```python
from build123d import *

# Parameters (mm, degrees)
PAD_DEPTH          = 9
SKETCH001_W        = 26.1
SKETCH001_H        = 34.4
POCKET_DEPTH       = 3
SKETCH002_R        = 22.22
PAD001_DEPTH       = 3
SKETCH003_R        = 24.44
PAD002_DEPTH       = 3
SKETCH004_R        = 26.6
PAD003_DEPTH       = 3
SKETCH005_R        = 28
PAD004_DEPTH       = 3
SKETCH006_R        = 29
PAD005_DEPTH       = 3
SKETCH007_R        = 29
PAD006_DEPTH       = 3
SKETCH008_R        = 29
PAD007_DEPTH       = 3
SKETCH009_W        = 17
SKETCH009_H        = 24
POCKET001_DEPTH    = 3
SKETCH010_W        = 16
SKETCH010_H        = 9
POCKET002_DEPTH    = 7
SKETCH011_W        = 20
SKETCH011_H        = 9
POCKET003_DEPTH    = 3
SKETCH012_R        = 1.25
POCKET004_DEPTH    = 270.433943
POLARPATTERN_COUNT = 6
SKETCH013_W        = 3
SKETCH013_H        = 38
POCKET005_DEPTH    = 3
SKETCH014_W        = 3
SKETCH014_H        = 6
POCKET006_DEPTH    = 6
SKETCH015_W        = 10.05
SKETCH015_H        = 6
POCKET007_DEPTH    = 3
FILLET_R           = 4


with BuildPart() as part:
    # Sketch → Pad (new body)
    with BuildSketch(Plane.XY):
        Polygon((44, 0), (22, 38.105118), (-22, 38.105118), (-44, 0), (-22, -38.105118), (22, -38.105118), align=None)
    extrude(amount=PAD_DEPTH)

    # Sketch001 (on Face8 of Pad) → Pocket (cut)
    with BuildSketch(Plane.XY.offset(9)):
        with Locations((0, -13.905118)):
            Rectangle(SKETCH001_W, SKETCH001_H)
    extrude(amount=-POCKET_DEPTH, mode=Mode.SUBTRACT)

    # Sketch002 (on Face5 of Pocket) → Pad001 (join)
    with BuildSketch(Plane.XY.offset(9)):
        Polygon((22, 38.105118), (-22, 38.105118), (-44, 0), (-22, -38.105118), (22, -38.105118), (44, 0), align=None)
        Circle(SKETCH002_R, mode=Mode.SUBTRACT)
    extrude(amount=PAD001_DEPTH)

    # Sketch003 (on Face14 of Pad001) → Pad002 (join)
    with BuildSketch(Plane.XY.offset(12)):
        Polygon((40, 0), (20, 34.641016), (-20, 34.641016), (-40, 0), (-20, -34.641016), (20, -34.641016), align=None)
        Circle(SKETCH003_R, mode=Mode.SUBTRACT)
    extrude(amount=PAD002_DEPTH)

    # Sketch004 (on Face21 of Pad002) → Pad003 (join)
    with BuildSketch(Plane.XY.offset(15)):
        Polygon((41, 0), (20.5, 35.507042), (-20.5, 35.507042), (-41, 0), (-20.5, -35.507042), (20.5, -35.507042), align=None)
        Circle(SKETCH004_R, mode=Mode.SUBTRACT)
    extrude(amount=PAD003_DEPTH)

    # Sketch005 (on Face28 of Pad003) → Pad004 (join)
    with BuildSketch(Plane.XY.offset(18)):
        Polygon((19, 32.908965), (-19, 32.908965), (-38, 0), (-19, -32.908965), (19, -32.908965), (38, 0), align=None)
        Circle(SKETCH005_R, mode=Mode.SUBTRACT)
    extrude(amount=PAD004_DEPTH)

    # Sketch006 (on Face35 of Pad004) → Pad005 (join)
    with BuildSketch(Plane.XY.offset(21)):
        Polygon((39, 0), (19.5, 33.774991), (-19.5, 33.774991), (-39, 0), (-19.5, -33.774991), (19.5, -33.774991), align=None)
        Circle(SKETCH006_R, mode=Mode.SUBTRACT)
    extrude(amount=PAD005_DEPTH)

    # Sketch007 (on Face42 of Pad005) → Pad006 (join)
    with BuildSketch(Plane.XY.offset(24)):
        Polygon((36, 0), (18, 31.176915), (-18, 31.176915), (-36, 0), (-18, -31.176915), (18, -31.176915), align=None)
        Circle(SKETCH007_R, mode=Mode.SUBTRACT)
    extrude(amount=PAD006_DEPTH)

    # Sketch008 (on Face49 of Pad006) → Pad007 (join)
    with BuildSketch(Plane.XY.offset(27)):
        Polygon((37, 0), (18.5, 32.04294), (-18.5, 32.04294), (-37, 0), (-18.5, -32.04294), (18.5, -32.04294), align=None)
        Circle(SKETCH008_R, mode=Mode.SUBTRACT)
    extrude(amount=PAD007_DEPTH)

    # Sketch009 (on Face74 of Pad007) → Pocket001 (cut)
    with BuildSketch(Plane.XY.offset(6)):
        with Locations((0, -8.705118)):
            Rectangle(SKETCH009_W, SKETCH009_H)
    extrude(amount=-POCKET001_DEPTH, mode=Mode.SUBTRACT)

    # Sketch010 (on Face12 of Pocket001) → Pocket002 (cut)
    with BuildSketch(Plane.XZ.offset(38.105118)):
        with Locations((0, 7.5)):
            Rectangle(SKETCH010_W, SKETCH010_H)
    extrude(amount=-POCKET002_DEPTH, mode=Mode.SUBTRACT)

    # Sketch011 (on Face40 of Pocket002) → Pocket003 (cut)
    with BuildSketch(Plane.XY.offset(9)):
        with Locations((0, 17.72)):
            Rectangle(SKETCH011_W, SKETCH011_H)
    extrude(amount=-POCKET003_DEPTH, mode=Mode.SUBTRACT)

    # Sketch012 (on Face93 of Pocket003) → Pocket004 (cut, through all)
    with BuildSketch(Plane.XY.offset(30)):
        with Locations((-32.33, 0)):
            Circle(SKETCH012_R)
    pocket004 = extrude(amount=-POCKET004_DEPTH, mode=Mode.SUBTRACT)

    # PolarPattern: Pocket004 ×6 about axis
    polarpattern_axis = Axis((0, 0, 30), (0, 0, 1))
    for i in range(1, POLARPATTERN_COUNT):
        add(pocket004.rotate(polarpattern_axis, i * 360 / POLARPATTERN_COUNT), mode=Mode.SUBTRACT)

    # Sketch013 (on Face45 of PolarPattern) → Pocket005 (cut)
    with BuildSketch(Plane.XY.offset(6)):
        with Locations((-11.55, -12.105118)):
            Rectangle(SKETCH013_W, SKETCH013_H)
    extrude(amount=-POCKET005_DEPTH, mode=Mode.SUBTRACT)

    # Sketch014 (on Face58 of Pocket005) → Pocket006 (cut)
    with BuildSketch(Plane.XY.offset(9)):
        with Locations((-11.55, 6.294882)):
            Rectangle(SKETCH014_W, SKETCH014_H)
    extrude(amount=-POCKET006_DEPTH, mode=Mode.SUBTRACT)

    # Sketch015 (on Face58 of Pocket006) → Pocket007 (cut)
    with BuildSketch(Plane.XY.offset(9)):
        with Locations((-5.025, 6.294882)):
            Rectangle(SKETCH015_W, SKETCH015_H)
    extrude(amount=-POCKET007_DEPTH, mode=Mode.SUBTRACT)

    # Fillet
    fillet_edges = [part.edges().sort_by_distance(p)[0] for p in [
        (22, -38.105118, 4.5),
        (44, 0, 4.5),
        (22, 38.105118, 4.5),
        (-22, 38.105118, 4.5),
        (-44, 0, 4.5),
        (-22, -38.105118, 4.5),
    ]]
    fillet(fillet_edges, radius=FILLET_R)


solid = part.part
```
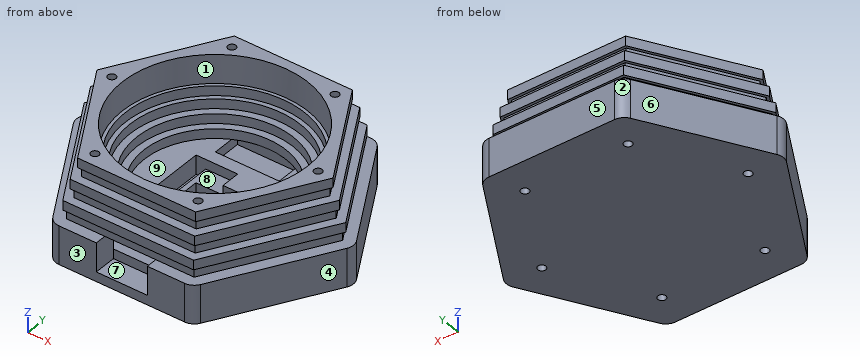
Check sheet for the modelled part. Datum: model origin and axes. Units: mm. Face numbers are marked on the shaded views. A direction names the side the tool comes from. Round coordinates to 2 decimals unless told otherwise and drop trailing zeros. Order: outer loops, then holes, each group sorted by start corner. A loop starts at its lowest first (then second) coordinate and runs counter-clockwise, first axis right, second up. Notation, with made-up numbers: (62.5, -29.75) - (111.5, -29.75) arc R36 ccw to (111.5, 4.25) - close; hole circle Ø9 at (-31.5, 44.5). An arc over 180 degrees is marked (long way). Answer as CSV lines item,"result". Start each with the question number.
1) Section check B-B (z = 4). Give the number of separate pieces and of enclosed holes in the cut face, then the cut area to 3 significant figures.
2) Scan lines: probe 1 along Z at (x, y) = (-8, 32); probe 2 along Y at (x, z) = (15.5, 23.75) (3 decimals); probe 3 along Z at (x, y) = (9, -33). Record each from-to range of solid material in increasing order.
3) Section check D-D (x = -35). Record the cut outline in (y, z), then the cut area to 3 significant figures.
4) Draft check along X on the marked faces 1, 2, 3 and 4. Enter one of: +X half, -X half, draft (parallel to the pull), parting line (faces both ways), or undercut.
5) Section check C-C (z = 19). Record the cut outline in (x, y) (3 decimals), then the cut area to 3 significant figures.
6) Tool access check on the marked faces 5, 6, 7, 8 and 9. Record the directions out of +Z, -Z, +X, -X, +Y, -Y that give a thin tool (end or side, any length) a straight path to the whole face; none if there is none.
7) Depth check by flat-ended pin: pin 1 (6 mm diameter, centred on x = 29.5, z = 16, fed in from -Y); pin 2 (10 mm diameter, centred on y = -13.5, z = 12, fed in from -X); pin 3 (0.9 mm diameter, centred on x = -6.5, z = 13.5, fed in from +Y). Enter the tip coordinate at first touch or a pass-through.
Determined:
1,separate pieces,"1"
1,enclosed holes,"8"
1,area,"4,350 mm^2"
2,probe 1,"0 to 24, 27 to 30"
2,probe 2,"-33.775 to -29.057, -26.94 to -24.51, 24.51 to 26.94, 29.057 to 33.775"
2,probe 3,"0 to 18, 21 to 24"
3,outline,"(-15.59, 0) - (15.59, 0) - (15.59, 12) - (8.66, 12) - (8.66, 15) - (10.39, 15) - (10.39, 18) - (5.2, 18) - (5.2, 21) - (6.93, 21) - (6.93, 24) - (1.73, 24) - (1.73, 27) - (3.46, 27) - (3.46, 30) - (-3.46, 30) - (-3.46, 27) - (-1.73, 27) - (-1.73, 24) - (-6.93, 24) - (-6.93, 21) - (-5.2, 21) - (-5.2, 18) - (-10.39, 18) - (-10.39, 15) - (-8.66, 15) - (-8.66, 12) - (-15.59, 12) - close"
3,area,"592 mm^2"
4,face 1,"undercut"
4,face 2,"-X half"
4,face 3,"draft"
4,face 4,"+X half"
5,outline,"(-38, 0) - (-19, -32.909) - (19, -32.909) - (38, 0) - (19, 32.909) - (-19, 32.909) - close; hole circle Ø2.5 at (-32.33, 0); hole circle Ø56 at (0, 0); hole circle Ø2.5 at (-16.165, -27.999); hole circle Ø2.5 at (-16.165, 27.999); hole circle Ø2.5 at (16.165, -27.999); hole circle Ø2.5 at (16.165, 27.999); hole circle Ø2.5 at (32.33, 0)"
5,area,"1,260 mm^2"
6,face 5,"+Z, -Z, +X, -X, +Y"
6,face 6,"+Z, -Z, -X, +Y"
6,face 7,"-Y"
6,face 8,"none"
6,face 9,"+Z"
7,pin 1,"y = -25.11"
7,pin 2,"x = -39.09"
7,pin 3,"y = 34.64"
